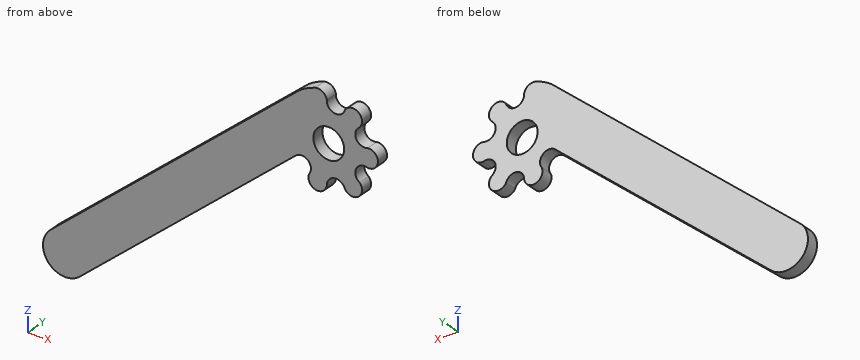
from build123d import *

# Parameters (mm, degrees)
EXTRUDE_1_DEPTH     = 2
SKETCH_2_R          = 2.5
CUT_EXTRUDE_1_DEPTH = 59.113082246


with BuildPart() as part:
    # Эскиз1 → Бобышка-Вытянуть1 (new body)
    with BuildSketch(Plane(origin=(0, 0, 0), x_dir=(1, 0, 0), z_dir=(0, 1, 0))):
        with BuildLine():
            Line((-5.373970273, 3.656561705), (-40.455802455, 34.00041309))
            ThreePointArc((-40.455802455, 34.00041309), (-45.556108034, 33.631060436), (-45.18675538, 28.530754857))
            Line((-45.18675538, 28.530754857), (-4.813797954, -6.389628256))
            ThreePointArc((-4.813797954, -6.389628256), (-3.570215935, -7.159159041), (-2.207328799, -7.689453789))
            ThreePointArc((-2.207328799, -7.689453789), (-0.992008234, -7.515625856), (-0.313557112, -6.492432667))
            ThreePointArc((-0.313557112, -6.492432667), (0.909859751, -4.914690841), (2.617012816, -5.949894446))
            ThreePointArc((2.617012816, -5.949894446), (4.813797954, -6.389628256), (4.997119526, -4.156777171))
            ThreePointArc((4.997119526, -4.156777171), (4.474545709, -2.231241963), (6.326923077, -1.489981335))
            ThreePointArc((6.326923077, -1.489981335), (8, 0), (6.326923077, 1.489981335))
            ThreePointArc((6.326923077, 1.489981335), (4.474545709, 2.231241963), (4.997119526, 4.156777171))
            ThreePointArc((4.997119526, 4.156777171), (4.813797954, 6.389628256), (2.617012816, 5.949894446))
            ThreePointArc((2.617012816, 5.949894446), (0.910344036, 4.916428962), (-0.31314214, 6.492452695))
            ThreePointArc((-0.31314214, 6.492452695), (-2.206837314, 7.689594857), (-3.177480342, 5.670416094))
            ThreePointArc((-3.177480342, 5.670416094), (-3.378992644, 3.685431957), (-5.373970273, 3.656561705))
        make_face()
    extrude(amount=EXTRUDE_1_DEPTH)

    # Эскиз2 → Вырез-Вытянуть1 (cut, through all)
    with BuildSketch(Plane(origin=(0, 2, 0), x_dir=(1, 0, 0), z_dir=(0, 1, 0))):
        with Locations(Location((0, 0, 0), (0, 0, 270))):
            Circle(SKETCH_2_R)
    extrude(amount=-CUT_EXTRUDE_1_DEPTH, mode=Mode.SUBTRACT)


solid = part.part
The model under review builds one solid part; all positions refer to its coordinate system, in mm. Coordinates: 2 decimals unless noted, no trailing zeros. Write each loop counter-clockwise with the first axis right and the second up, starting at its lowest first coordinate (ties: lowest second). Pieces come first, ordered by that corner, then holes. Notation, with made-up numbers: (67.25, 17) - (98.25, 17) arc R15 cw to (98.25, 42) - close; hole circle Ø8 at (41, 77.5). An arc over 180 degrees is marked (long way). Answer as CSV lines item,"result".
(1) We need section C-C (x = -8.5). Give the boundary of the cut face in (y, z).
Data:
outline,"(0, -6.36) - (2, -6.36) - (2, 3.2) - (0, 3.2) - close"
(2) For line 1 along X through (y, z) = (1.8, -6); line 2 along X through (y, z) = (1, 0); line 3 along Z through (x, y) = (-26, 1.2), list the stretches that pass through material, from the lowest coordinate up. Write a range as [from, to].
Data:
line 1,"x = [-19.14, -8.08], [-3.27, -0.26], [2.65, 5.17]"
line 2,"x = [-12.2, -2.5], [2.5, 8]"
line 3,"z = [-21.5, -11.94]"
(3) We need section A-A (y = 1.5). Give the boundary of the cut face in (x, z).
Data:
outline,"(-45.19, -28.53) arc R3.62 ccw to (-40.46, -34) - (-5.37, -3.66) arc R1.5 cw to (-3.18, -5.67) arc R1.5 ccw (long way) to (-0.31, -6.49) arc R1.5 cw to (2.62, -5.95) arc R1.5 ccw (long way) to (5, -4.16) arc R1.5 cw to (6.33, -1.49) arc R1.5 ccw (long way) to (6.33, 1.49) arc R1.5 cw to (5, 4.16) arc R1.5 ccw (long way) to (2.62, 5.95) arc R1.5 cw to (-0.31, 6.49) arc R1.5 ccw to (-2.21, 7.69) arc R8 ccw to (-4.81, 6.39) - close; hole circle Ø5 at (0, 0)"
(4) We need section B-B (z = 0). Give the boundary of the cut face in (x, y).
Data:
outline,"(-12.2, 0) - (-2.5, 0) - (-2.5, 2) - (-12.2, 2) - close; (2.5, 0) - (8, 0) - (8, 2) - (2.5, 2) - close"
(5) We need section D-D (z = -11). Give the boundary of the cut face in (x, y).
Data:
outline,"(-24.92, 0) - (-13.86, 0) - (-13.86, 2) - (-24.92, 2) - close"
